Part model, mm, in its own coordinate system. A direction names the side the tool comes from. Round coordinates to 2 decimals unless told otherwise and drop trailing zeros. Write each loop counter-clockwise with the first axis right and the second up, starting at its lowest first coordinate (ties: lowest second). Pieces come first, ordered by that corner, then holes.
1) Saw through at D-D on y = -2.25. Write the cut outline in (x, z).
2) Which spindle directions (+Z, -Z, +X, -X, +Y, -Y) get a long thin tool onto all of the face, cutting with end or side? Do faces 4 (the flat face through (-11, 0, 3)), 5 (the flat face through (-9, -5, 9)). Say none if no direction does.
3) Saw through at C-C on y = 13.5. Write the cut outline in (x, z).
4) Saw through at A-A on x = 0. Write the cut outline in (y, z), and give its area (3 significant figures).
5) Flat gauge pins, fed straight in: pin 1 (3 mm diameter, centred on x = -2, z = 11, fed in from -Y); pin 2 (20 mm diameter, centred on x = 2, z = -8, fed in from +Y); pin 3 (3 mm diameter, centred on x = -10.5, y = 6.5, fed in from +Z); pin 4 (1 mm diameter, centred on x = 17, y = 6, fed in from +Z). Where does each tip first touch, or does it go through?
6) Saw through at B-B on y = 9. Write the cut outline in (x, z), and give its area (3 significant figures).
7) Drill centre lines: L1, parallel to X at y = 10.5, z = 0; L2, parallel to Z at x = 9.5, y = 1.5; L3, parallel to X at y = 4.75, z = 12. Where is each one in solid material? Low to high.
8) Pull direction X, two halves, no side cores. Call faces 1 (the cylindrical face through (-13.417, 5.86, -17.498)), 2 (the flat face through (-9.7, 16, 19.5)), 3 (the cylindrical face through (-15.925, 5.423, 8.283)): +X half, -X half, draft (parallel to the pull), parting line (faces both ways), or undercut.
```python
from build123d import *

# Parameters (mm, degrees)
CROQUIS1_R              = 22.05
CROQUIS1_R_2            = 20.05
SALIENTE_EXTRUIR1_DEPTH = 16
CROQUIS1_4_R            = 17.95
CROQUIS1_4_R_2          = 16.2
SALIENTE_EXTRUIR2_DEPTH = 12.5
SALIENTE_EXTRUIR4_START = -5
CROQUIS1_6_R            = 22.05
CROQUIS1_6_R_2          = 20.05
CROQUIS1_6_R_3          = 17.95
CROQUIS1_6_R_4          = 16.2
SALIENTE_EXTRUIR4_DEPTH = 5
CORTAR_EXTRUIR1_REACH   = 39.595
CROQUIS4_R              = 11.05
CROQUIS4_R_2            = 1.25
REDONDEO1_R             = 1
REDONDEO2_R             = 1.5
REDONDEO3_R             = 1


with BuildPart() as part:
    # Croquis1 → Saliente-Extruir1 (new body)
    with BuildSketch(Plane(origin=(0, 0, 0), x_dir=(1, 0, 0), z_dir=(0, 1, 0))):
        with Locations(Location((0, 0, 0), (0, 0, 270))):
            Circle(CROQUIS1_R)
        with Locations(Location((0, 0, 0), (0, 0, 270))):
            Circle(CROQUIS1_R_2, mode=Mode.SUBTRACT)
    extrude(amount=SALIENTE_EXTRUIR1_DEPTH)



with BuildPart() as body_2:
    # Croquis1<4> → Saliente-Extruir2 (new body)
    with BuildSketch(Plane(origin=(0, 0, 0), x_dir=(1, 0, 0), z_dir=(0, 1, 0))):
        with Locations(Location((0, 0, 0), (0, 0, 270))):
            Circle(CROQUIS1_4_R)
        with Locations(Location((0, 0, 0), (0, 0, 270))):
            Circle(CROQUIS1_4_R_2, mode=Mode.SUBTRACT)
    extrude(amount=SALIENTE_EXTRUIR2_DEPTH)


with BuildPart() as part_1:
    add(part.part)

    add(body_2.part)  # Saliente-Extruir4 merges body 2
    # Croquis1<6> → Saliente-Extruir4 (add)
    # profile 1 of 4: a face of its own
    with BuildSketch(Plane(origin=(0, 0, 0), x_dir=(1, 0, 0), z_dir=(0, 1, 0)).offset(SALIENTE_EXTRUIR4_START)):
        with Locations(Location((0, 0, 0), (0, 0, 270))):
            Circle(CROQUIS1_6_R)
        with Locations(Location((0, 0, 0), (0, 0, 270))):
            Circle(CROQUIS1_6_R_2, mode=Mode.SUBTRACT)
    # profile 2 of 4: a face of its own
    with BuildSketch(Plane(origin=(0, 0, 0), x_dir=(1, 0, 0), z_dir=(0, 1, 0)).offset(SALIENTE_EXTRUIR4_START)):
        with Locations(Location((0, 0, 0), (0, 0, 270))):
            Circle(CROQUIS1_6_R_2)
        with Locations(Location((0, 0, 0), (0, 0, 270))):
            Circle(CROQUIS1_6_R_3, mode=Mode.SUBTRACT)
    # profile 3 of 4: a face of its own
    with BuildSketch(Plane(origin=(0, 0, 0), x_dir=(1, 0, 0), z_dir=(0, 1, 0)).offset(SALIENTE_EXTRUIR4_START)):
        with Locations(Location((0, 0, 0), (0, 0, 270))):
            Circle(CROQUIS1_6_R_3)
        with Locations(Location((0, 0, 0), (0, 0, 270))):
            Circle(CROQUIS1_6_R_4, mode=Mode.SUBTRACT)
    # profile 4 of 4: a face of its own
    with BuildSketch(Plane(origin=(0, 0, 0), x_dir=(1, 0, 0), z_dir=(0, 1, 0)).offset(SALIENTE_EXTRUIR4_START)):
        with Locations(Location((0, 0, 0), (0, 0, 270))):
            Circle(CROQUIS1_6_R_4)
    extrude(amount=SALIENTE_EXTRUIR4_DEPTH)

    # Croquis4 → Cortar-Extruir1 (cut, up to next)
    with BuildSketch(Plane.XZ.offset(5), mode=Mode.PRIVATE) as cortar_extruir1_sk1:
        with Locations(Location((0, 0, 0), (0, 0, 270))):
            Circle(CROQUIS4_R)
    cortar_extruir1_tool1 = extrude(cortar_extruir1_sk1.sketch, amount=-CORTAR_EXTRUIR1_REACH, mode=Mode.PRIVATE) & part_1.part
    # Croquis4 → Cortar-Extruir1 (cut, up to next)
    with BuildSketch(Plane.XZ.offset(5), mode=Mode.PRIVATE) as cortar_extruir1_sk2:
        with Locations(Location((9.5, 12, 0), (0, 0, 270))):
            Circle(CROQUIS4_R_2)
    cortar_extruir1_tool2 = extrude(cortar_extruir1_sk2.sketch, amount=-CORTAR_EXTRUIR1_REACH, mode=Mode.PRIVATE) & part_1.part
    # Croquis4 → Cortar-Extruir1 (cut, up to next)
    with BuildSketch(Plane.XZ.offset(5), mode=Mode.PRIVATE) as cortar_extruir1_sk3:
        with Locations(Location((-9.5, -12, 0), (0, 0, 270))):
            Circle(CROQUIS4_R_2)
    cortar_extruir1_tool3 = extrude(cortar_extruir1_sk3.sketch, amount=-CORTAR_EXTRUIR1_REACH, mode=Mode.PRIVATE) & part_1.part
    add(cortar_extruir1_tool1.solids().sort_by_distance((0, -5, 0))[0], mode=Mode.SUBTRACT)
    add(cortar_extruir1_tool2.solids().sort_by_distance((9.5, -5, 12))[0], mode=Mode.SUBTRACT)
    add(cortar_extruir1_tool3.solids().sort_by_distance((-9.5, -5, -12))[0], mode=Mode.SUBTRACT)

    # Redondeo1
    redondeo1_edges = [part_1.edges().sort_by_distance(p)[0] for p in [
        (0, -5, 11.05),
    ]]
    fillet(redondeo1_edges, radius=REDONDEO1_R)

    # Redondeo2
    # the kernel refuses this fillet: 1.5 mm, written as the material it takes off along each edge
    with BuildSketch(Plane(origin=(0, 12.5, 0), x_dir=(0, 0, 1), z_dir=(-1, 0, 0))) as redondeo2_piece_1:
        with BuildLine():
            CenterArc((17.95 - REDONDEO2_R, -REDONDEO2_R), REDONDEO2_R, 0, 90)
            Line((17.95, -REDONDEO2_R), (17.95, 0))
            Line((17.95, 0), (17.95 - REDONDEO2_R, 0))
        make_face()
    revolve(axis=Axis((0, 12.5, 0), (0, 1, 0)), mode=Mode.SUBTRACT)
    with BuildSketch(Plane(origin=(0, 16, 0), x_dir=(0, 0, 1), z_dir=(-1, 0, 0))) as redondeo2_piece_2:
        with BuildLine():
            CenterArc((20.05 + REDONDEO2_R, -REDONDEO2_R), REDONDEO2_R, 90, 90)
            Line((20.05, -REDONDEO2_R), (20.05, 0))
            Line((20.05, 0), (20.05 + REDONDEO2_R, 0))
        make_face()
    revolve(axis=Axis((0, 16, 0), (0, 1, 0)), mode=Mode.SUBTRACT)

    # Redondeo3
    redondeo3_edges = [part_1.edges().sort_by_distance(p)[0] for p in [
        (0, -5, -22.05),
    ]]
    fillet(redondeo3_edges, radius=REDONDEO3_R)


solid = part_1.part
```
Completed:
1. outline: circle Ø44.1 at (0, 0); hole circle Ø22.1 at (0, 0); hole circle Ø2.5 at (-9.5, -12); hole circle Ø2.5 at (9.5, 12)
2. face 4: +Y
2. face 5: +Z, -Z, +X, -X, -Y
3. outline: circle Ø44.1 at (0, 0); hole circle Ø40.1 at (0, 0)
4. outline: (-5, -21.05) arc R1 ccw to (-4, -22.05) - (16, -22.05) - (16, -21.55) arc R1.5 ccw to (14.5, -20.05) - (0, -20.05) - (0, -17.95) - (11, -17.95) arc R1.5 ccw to (12.5, -16.45) - (12.5, -16.2) - (0, -16.2) - (0, -11.05) - (-4, -11.05) arc R1 ccw to (-5, -12.05) - close; (-5, 12.05) arc R1 ccw to (-4, 11.05) - (0, 11.05) - (0, 16.2) - (12.5, 16.2) - (12.5, 16.45) arc R1.5 ccw to (11, 17.95) - (0, 17.95) - (0, 20.05) - (14.5, 20.05) arc R1.5 ccw to (16, 21.55) - (16, 22.05) - (-4, 22.05) arc R1 ccw to (-5, 21.05) - close
4. area: 215 mm2
5. pin 1: stops at y = -5
5. pin 2: stops at y = 12.5
5. pin 3: stops at z = 20.13
5. pin 4: stops at z = 14.63
6. outline: circle Ø44.1 at (0, 0); circle Ø35.9 at (0, 0); hole circle Ø40.1 at (0, 0); hole (-10.74, -12.12) arc R1.25 ccw to (-9.34, -13.24) arc R16.2 ccw to (10.74, 12.12) arc R1.25 ccw to (9.34, 13.24) arc R16.2 ccw to start
6. area: 451 mm2
7. L1: x = -22.05 to -20.05, -17.95 to -16.2, 16.2 to 17.95, 20.05 to 22.05
7. L2: z = -19.9 to -17.66, -15.23 to -13.12, 13.25 to 15.23, 17.66 to 19.9
7. L3: x = -18.5 to -16.06, -13.35 to -10.88, 10.88 to 13.35, 16.06 to 18.5
8. face 1: parting line
8. face 2: draft
8. face 3: undercut
